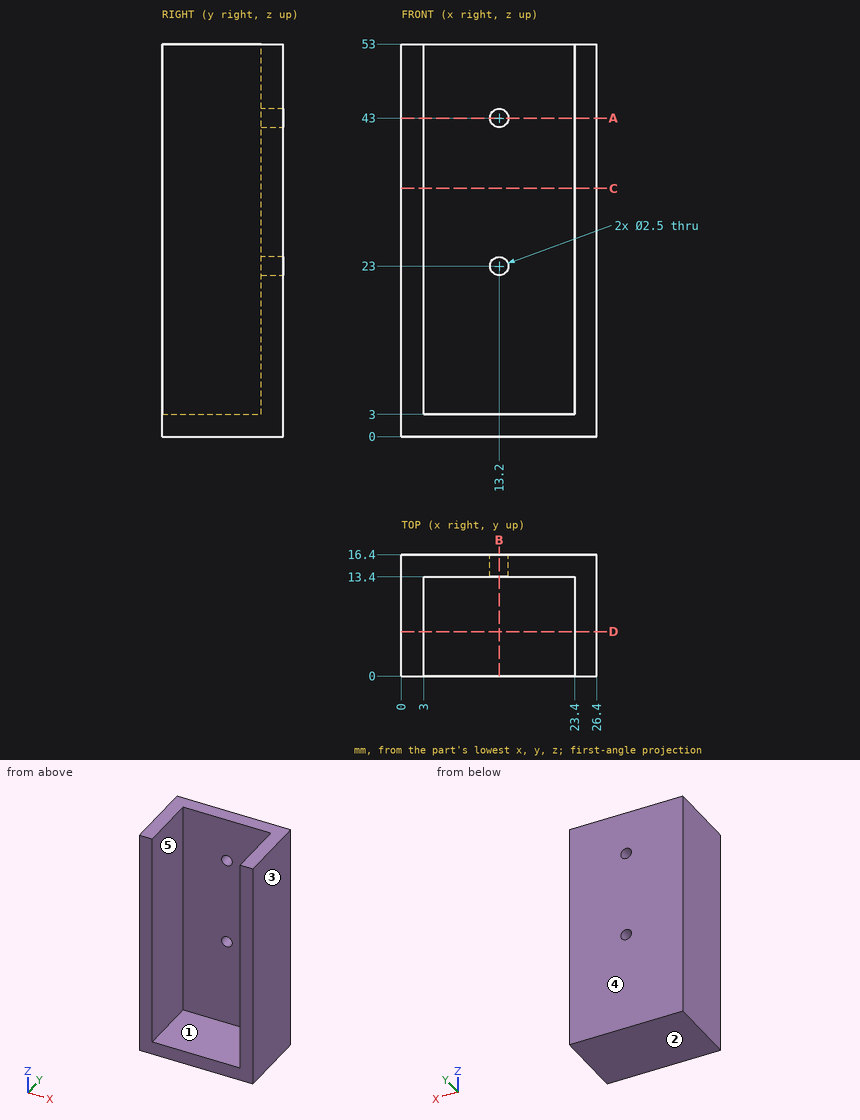
Verification items for this drawing (mm, ordinates from the low corner). A direction names the side the tool comes from. Round coordinates to 2 decimals unless told otherwise and drop trailing zeros. Order: outer loops, then holes, each group sorted by start corner. A loop starts at its lowest first (then second) coordinate and runs counter-clockwise, first axis right, second up. Notation, with made-up numbers: (73, 74.25) - (117, 74.25) arc R24 cw to (117, 108.25) - close; hole circle Ø5 at (51, 64.25). An arc over 180 degrees is marked (long way). Use CSV: the item, a comma, the result in double quotes.
(1) Section check D-D on y = 6. Record the boundary of the cut face in (x, z), and give its area (3 significant figures).
Entries:
outline,"(0, 0) - (26.4, 0) - (26.4, 53) - (23.4, 53) - (23.4, 3) - (3, 3) - (3, 53) - (0, 53) - close"
area,"379 mm^2"
(2) Section check B-B on x = 13.2. Record the boundary of the cut face in (y, z), and give its area (3 significant figures).
Entries:
outline,"(0, 0) - (16.4, 0) - (16.4, 21.75) - (13.4, 21.75) - (13.4, 3) - (0, 3) - close; (13.4, 24.25) - (16.4, 24.25) - (16.4, 41.75) - (13.4, 41.75) - close; (13.4, 44.25) - (16.4, 44.25) - (16.4, 53) - (13.4, 53) - close"
area,"184 mm^2"
(3) Access from +Z, -Z, +X, -X, +Y, -Y to the whole of each face (thin tool, end or side, straight path). Record for the marked faces 4 and 5.
Entries:
face 4,"+Z, -Z, +X, -X, +Y"
face 5,"+Z, -Y"
(4) Section check A-A on z = 43. Record the boundary of the cut face in (x, y).
Entries:
outline,"(0, 0) - (3, 0) - (3, 13.4) - (11.95, 13.4) - (11.95, 16.4) - (0, 16.4) - close; (14.45, 13.4) - (23.4, 13.4) - (23.4, 0) - (26.4, 0) - (26.4, 16.4) - (14.45, 16.4) - close"
(5) Thickness scan on probe 1 along X at (y, z) = (14.95, 23); probe 2 along X at (y, z) = (1.5, 21.5); probe 3 along Y at (x, z) = (4.25, 37). Record the ranges inside material, lowest first. Write a range as from..to.
Entries:
probe 1,"0..11.95, 14.45..26.4"
probe 2,"0..3, 23.4..26.4"
probe 3,"13.4..16.4"
(6) Section check C-C on z = 33.5. Record the boundary of the cut face in (x, y).
Entries:
outline,"(0, 0) - (3, 0) - (3, 13.4) - (23.4, 13.4) - (23.4, 0) - (26.4, 0) - (26.4, 16.4) - (0, 16.4) - close"
(7) Gauge pin test, flat ends, axial feed: pin 1 Ø2 at (x, z) = (13.2, 43) entering from +Y; pin 2 Ø5 at (x, y) = (16.5, 11.5) entering from +Z; pin 3 Ø10 at (x, z) = (12, 18.5) entering from -Y; pin 4 Ø6.5 at (x, y) = (9.5, 9) entering from +Z. Record the tip position at first contact, or that the pin passes through.
Entries:
pin 1,"through"
pin 2,"z = 53"
pin 3,"y = 13.4"
pin 4,"z = 3"
(8) Mould release check, pull along X, two halves, no side actions. Record for the marked faces 1, 2 and 3: released by +X, released by -X, zero draft, split by the parting line, or undercut.
Entries:
face 1,"undercut"
face 2,"zero draft"
face 3,"released by +X"
